The listing builds one solid part. Answer for the finished solid, in the listing's coordinates (mm). A direction names the side the tool comes from. Round coordinates to 2 decimals unless told otherwise and drop trailing zeros. Order: outer loops, then holes, each group sorted by start corner. A loop starts at its lowest first (then second) coordinate and runs counter-clockwise, first axis right, second up. Notation, with made-up numbers: (18.25, -11.5) -> (59.25, -11.5) arc R19 ccw to (59.25, -5.5) -> close; hole circle Ø10 at (-22, 18). An arc over 180 degrees is marked (long way). Return JSON: item names as keys, results as strings. Group by question number.
(1) The part is cut by section D-D (x = -3). Determine the outline of the cut face in (y, z).
(2) Which of the six approach directions +Z, -Z, +X, -X, +Y, -Y give full straight-line access (tool end or side, diameter ignored) to faces 5 (the face through (-1.5, 1, 0)), 6 (the face through (-2, 0, -2))?
(3) The part is cut by section A-A (y = 0.5). Determine the outline of the cut face in (x, z).
(4) The part is cut by section C-C (y = -31.5). Determine the outline of the cut face in (x, z).
(5) Each of these flat-tipped pins is pushed along its axis until it touches: pin 1 (0.5 mm diameter, centred on y = 1.5, z = 0, fed in from +X); pin 2 (2 mm diameter, centred on y = -9, z = 0, fed in from +X); pin 3 (2 mm diameter, centred on x = -1.5, y = -22, fed in from -Z). Where does it stop, or does it pass through?
(6) Consider line 1 (X direction, y = -13, z = 2); line 2 (Z direction, x = 0, y = -24); line 3 (Y direction, x = 2.5, z = -3.5). Determine where each line is inside the solid, lowest interval first. Write a range as [from, to].
(7) The part is cut by section B-B (z = 0). Determine the outline of the cut face in (x, y), plus the area to 3 significant figures.
(8) Determine the mould class of faces 1 (the face through (0.74, 1.273, 1.305)), 2 (the face through (0.761, 1.273, -1.293)), 3 (the face through (-0.54, -17.26, -2.44)), 4 (the face through (0, -35, 0)) for opening direction X: +X half, -X half, draft (parallel to the pull), parting line (faces both ways), or undercut.
from build123d import *

# Parameters (mm, degrees)
CUT_EXTRUDE1_DEPTH = 10


with BuildPart() as part:
    # Sketch1 → Revolve1 (revolve)
    with BuildSketch(Plane.XY):
        with BuildLine():
            Line((0, 0), (0, -35))
            Line((0, -35), (2.5, -35))
            Line((2.5, -35), (2.5, 0))
            Line((2.5, 0), (4.65, 0))
            ThreePointArc((4.65, 0), (2.713968497, 2.045965539), (0, 2.8))
            Line((0, 2.8), (0, 0))
        make_face()
    revolve(axis=Axis((0, 0, 0), (0, -1, 0)))

    # Sketch2 → Cut-Extrude1 (cut)
    with BuildSketch(Plane(origin=(0, 0, 0), x_dir=(1, 0, 0), z_dir=(0, 1, 0))):
        Polygon((0, 1.732050808), (-1.5, 0.866025404), (-1.5, -0.866025404), (0, -1.732050808), (1.5, -0.866025404), (1.5, 0.866025404), align=None)
    extrude(amount=CUT_EXTRUDE1_DEPTH, mode=Mode.SUBTRACT)


solid = part.part
Answer below:
{
 "1": {"outline": "(0, -3.55) arc R4.32 ccw to (0, 3.55) -> close"},
 "2": {"face 5": "+Y", "face 6": "-Y"},
 "3": {"outline": "circle Ø8.7 at (0, 0); hole (-1.5, -0.87) -> (0, -1.73) -> (1.5, -0.87) -> (1.5, 0.87) -> (0, 1.73) -> (-1.5, 0.87) -> close"},
 "4": {"outline": "circle Ø5 at (0, 0)"},
 "5": {"pin 1": "stops at x = 3.73", "pin 2": "stops at x = 2.5", "pin 3": "stops at z = -2.45"},
 "6": {"line 1": "x = [-1.5, 1.5]", "line 2": "z = [-2.5, 2.5]", "line 3": "y = [0, 0.57]"},
 "7": {"outline": "(-4.65, 0) -> (-2.5, 0) -> (-2.5, -35) -> (2.5, -35) -> (2.5, 0) -> (4.65, 0) arc R5.26 ccw to (1.5, 2.58) -> (1.5, 0) -> (-1.5, 0) -> (-1.5, 2.58) arc R5.26 ccw to start", "area": "185 mm²"},
 "8": {"face 1": "undercut", "face 2": "undercut", "face 3": "parting line", "face 4": "draft"}
}
